Geometry: final body of the model. Coordinates: model frame, mm. A direction names the side the tool comes from. Round coordinates to 2 decimals unless told otherwise and drop trailing zeros. Loops run counter-clockwise (first coordinate to the right, second up) from the corner with the lowest first, then second, coordinate; pieces in that order, holes last. Notation, with made-up numbers: (57, 68.25) - (107, 68.25) arc R20 ccw to (107, 72.25) - close; hole circle Ø7 at (45.5, 83.5). An arc over 180 degrees is marked (long way). Answer as a JSON object with one key per item and string values. Group by question number.
Item 1: Draft query along Z for faces 1 (the face through (-1.338, 13.305, -6.027)), 2 (the face through (3, 8, 5)), 3 (the face through (5.4, 10, 5.4)). Return one class per face: released by +Z, released by -Z, zero draft, split by the parting line, or undercut.
Item 2: Section B-B (x = 0). Return the cut outline in (y, z), plus the area to 3 significant figures.
Item 3: Reachability of faces 4 (the face through (0, 12, 0)), 5 (the face through (-18.2, 0, 9.9)) from +Z, -Z, +X, -X, +Y, -Y: full face, straight path, thin tool, end or side. Return the list, or none.
Item 4: First-contact query: pin 1 (6 mm diameter, centred on x = 17.5, z = 1, fed in from +Y); pin 2 (20 mm diameter, centred on x = -6, z = -1.5, fed in from -Y); pin 3 (3 mm diameter, centred on x = -1.5, y = 3.5, fed in from -Z). Flat tips, straight axial feed; report the tip coordinate or a pass-through.
Item 5: Section C-C (y = 12.75). Return the cut outline in (x, z) (1 decimal).
Item 6: Section A-A (z = 0). Return the cut outline in (x, y).
Item 7: Line query: line 1 (X direction, y = 5.75, z = -2.5); line 2 (X direction, y = 3.75, z = -12.5); line 3 (Z direction, x = -13, y = 4.75). Output: solid intervals per line, ascending.
Autodesk Inventor part; units mm, degrees
ref_plane "YZ Plane" through (0, 0, 0) normal (1, 0, 0) x (0, 1, 0)
ref_plane "XZ Plane" through (0, 0, 0) normal (0, 1, 0) x (-1, 0, 0)
ref_plane "XY Plane" through (0, 0, 0) normal (0, 0, 1) x (1, 0, 0)
sketch "Sketch1" plane through (0, 0, 0) normal (0, 0, 1) x (1, 0, 0)
  line L0 (0, 0) -> (22.5, 0) construction
  line L1 (0, 0) -> (0, 10) construction
  line L2 (0, 10) -> (7, 10) construction
  line L3 (7, 10) -> (0, 10) construction
  line L4 (0, 10) -> (0, 14) construction
  line L5 (0, 14) -> (6, 14) construction
  line L6 (0, 10) -> (12.5, 10) construction
  line L7 (6, 14) -> (7, 10)
  line L8 (7, 10) -> (12.5, 10)
  line L9 (12.5, 10) -> (12.5, 10)
  line L10 (22.5, 0) -> (22.5, 0)
  arc A0 (22.5, 0) -> (12.5, 10) centre (12.5, 0) ccw
  line L11 (6, 14) -> (0, 14)
  point P0 (22.5, 10)
  dimension "d0" = 22.5
  dimension "d1" = 10
  dimension "d2" = 7
  dimension "d3" = 4
  dimension "d4" = 6
  dimension "d5" = 12.5
  dimension "d6" = 10
surface revolve "RevolutionSrf1" sketch "Sketch1" angle 360 about axis through (0, 0, 0) along (0, 1, 0) shown no curves L10 A0 L9 L8 L7 L11
thicken "Thicken1" operation new thickness 2 both sides no extend neighbours no toward (0, -1, 0) faces at (-0.7092, 14, -1.4219) (6.4729, 11.3333, 1.5954) (10.5456, 10, 0.9971) (22.181, 0.7473, 3.6048)
properties part number "cup"
Values:
{
 "1": {"face 1": "split by the parting line", "face 2": "undercut", "face 3": "zero draft"},
 "2": {"outline": "(0, -22.5) arc R10 ccw to (10, -12.5) - (10, -7) - (14, -6) - (14, 6) - (10, 7) - (10, 12.5) arc R10 ccw to (0, 22.5) - (0, 20.5) arc R8 cw to (8, 12.5) - (8, 5.44) - (12, 4.44) - (12, -4.44) - (8, -5.44) - (8, -12.5) arc R8 cw to (0, -20.5) - close", "area": "119 mm^2"},
 "3": {"face 4": "-Y", "face 5": "+Z, -Z, +X, -X, -Y"},
 "4": {"pin 1": "stops at y = 9.79", "pin 2": "stops at y = 7.1", "pin 3": "stops at z = -22.26"},
 "5": {"outline": "circle Ø12.6 at (0, 0)"},
 "6": {"outline": "(-22.5, 0) - (-20.5, 0) arc R8 cw to (-12.5, 8) - (-5.44, 8) - (-4.44, 12) - (4.44, 12) - (5.44, 8) - (12.5, 8) arc R8 cw to (20.5, 0) - (22.5, 0) arc R10 ccw to (12.5, 10) - (7, 10) - (6, 14) - (-6, 14) - (-7, 10) - (-12.5, 10) arc R10 ccw to start"},
 "7": {"line 1": "x = -20.53 to -17.89, 17.89 to 20.53", "line 2": "x = -17.82 to -15.05, 15.05 to 17.82", "line 3": "z = -16.87 to -13.77, 13.77 to 16.87"}
}
